Could you check a few things on this drawing? It's one solid part, dimensions in mm from its lowest x, y, z. Give positions to 0.01 mm unless a question says otherwise; leave off trailing zeros. Order: outer loops, then holes, each group sorted by start corner. A loop starts at its lowest first (then second) coordinate and runs counter-clockwise, first axis right, second up.
(1) Imagine slicing it at C-C, the plane x = 1150. Write out the boundary of the cut face in (y, z).
(2) Imagine slicing it at B-B, the plane z = 57. Write out the boundary of the cut face in (x, y), then the cut area to 3 significant figures.
(3) Imagine slicing it at D-D, the plane y = 634.5. Write out the boundary of the cut face in (x, z), then the cut area to 3 significant figures.
(4) Imagine slicing it at A-A, the plane y = 2000. Write out the boundary of the cut face in (x, z).
(5) If I drill on probe 1 along Y at (x, z) = (1150, 76); probe 2 along X at (y, z) = (2000, 79); probe 3 along X at (y, z) = (368.5, 65.5), over which ranges is the centre line in solid material (lowest first)?
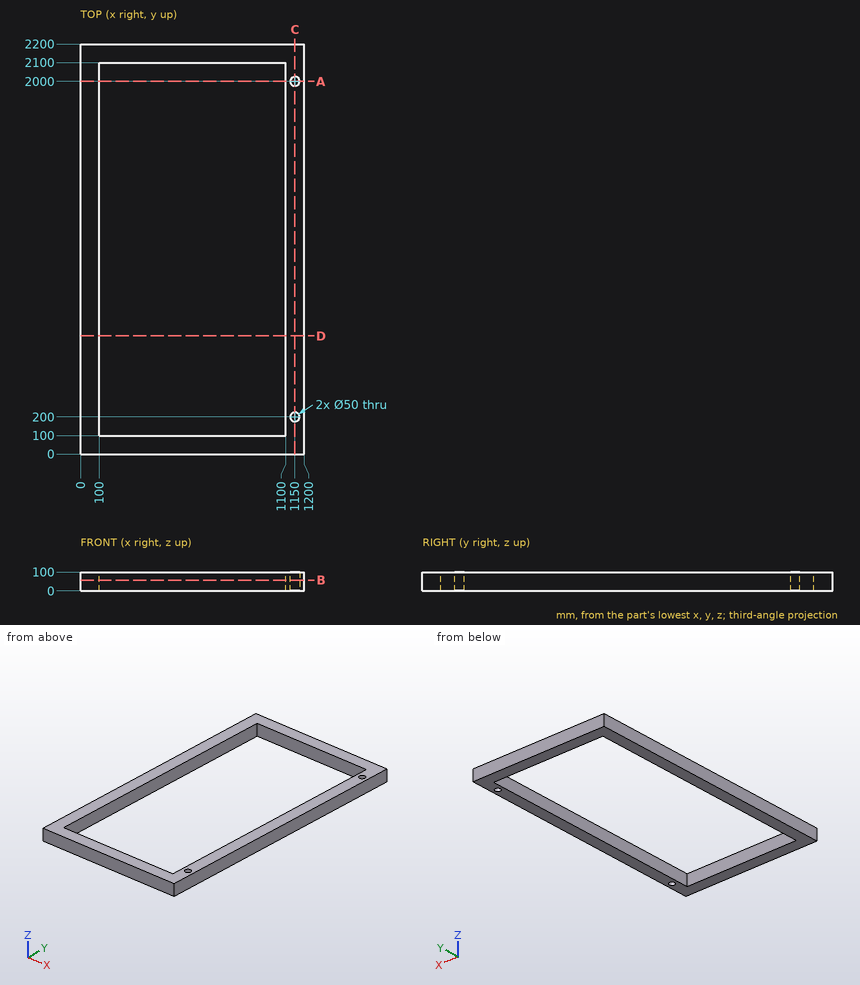
Answer block:
1. outline: (0, 0) - (175, 0) - (175, 100) - (0, 100) - close; (225, 0) - (1975, 0) - (1975, 100) - (225, 100) - close; (2025, 0) - (2200, 0) - (2200, 100) - (2025, 100) - close
2. outline: (0, 0) - (1200, 0) - (1200, 2200) - (0, 2200) - close; hole (100, 100) - (1100, 100) - (1100, 2100) - (100, 2100) - close; hole circle Ø50 at (1150, 200); hole circle Ø50 at (1150, 2000)
2. area: 636,000 mm2
3. outline: (0, 0) - (100, 0) - (100, 100) - (0, 100) - close; (1100, 0) - (1200, 0) - (1200, 100) - (1100, 100) - close
3. area: 20,000 mm2
4. outline: (0, 0) - (100, 0) - (100, 100) - (0, 100) - close; (1100, 0) - (1125, 0) - (1125, 100) - (1100, 100) - close; (1175, 0) - (1200, 0) - (1200, 100) - (1175, 100) - close
5. probe 1: y = 0 to 175, 225 to 1975, 2025 to 2200
5. probe 2: x = 0 to 100, 1100 to 1125, 1175 to 1200
5. probe 3: x = 0 to 100, 1100 to 1200
